Geometry: final body of the model. Coordinates: model frame, mm. A direction names the side the tool comes from. Coordinates: 2 decimals unless noted, no trailing zeros. Order: outer loops, then holes, each group sorted by start corner. A loop starts at its lowest first (then second) coordinate and runs counter-clockwise, first axis right, second up. Notation, with made-up numbers: (8, 86) -> (54, 86) arc R15 cw to (54, 90) -> close; hole circle Ø2 at (0.5, -33.5). An arc over 180 degrees is marked (long way). Use one line per item in the form item = value.
```python
from build123d import *

# Parameters (mm, degrees)
SKETCH1_W           = 150
SKETCH1_H           = 140
SKETCH1_R           = 2.85
SKETCH1_R_2         = 4
BOSS_EXTRUDE1_DEPTH = 5
SKETCH2_W           = 32
SKETCH2_H           = 18
SKETCH2_R           = 4
BOSS_EXTRUDE2_DEPTH = 5


with BuildPart() as part:
    # Sketch1 → Boss-Extrude1 (new body)
    with BuildSketch(Plane(origin=(0, 0, 0), x_dir=(1, 0, 0), z_dir=(0, 1, 0))):
        with Locations((-0.545997502, 48.457242913)):
            Rectangle(SKETCH1_W, SKETCH1_H)
        with Locations(Location((-65.545997502, 108.457242913, 0), (0, 0, 270))):
            Circle(SKETCH1_R, mode=Mode.SUBTRACT)
        with Locations(Location((64.454002498, 108.457242913, 0), (0, 0, 270))):
            Circle(SKETCH1_R, mode=Mode.SUBTRACT)
        with Locations(Location((64.454002498, -11.542757087, 0), (0, 0, 270))):
            Circle(SKETCH1_R, mode=Mode.SUBTRACT)
        with Locations(Location((-65.545997502, -11.542757087, 0), (0, 0, 270))):
            Circle(SKETCH1_R, mode=Mode.SUBTRACT)
        with Locations(Location((-11.545997502, 48.457242913, 0), (0, 0, 270))):
            Circle(SKETCH1_R_2, mode=Mode.SUBTRACT)
        with Locations(Location((-0.545997502, 48.457242913, 0), (0, 0, 270))):
            Circle(SKETCH1_R_2, mode=Mode.SUBTRACT)
        with Locations(Location((10.454002498, 48.457242913, 0), (0, 0, 270))):
            Circle(SKETCH1_R_2, mode=Mode.SUBTRACT)
    extrude(amount=BOSS_EXTRUDE1_DEPTH)

    # Sketch2 → Boss-Extrude2 (add)
    with BuildSketch(Plane(origin=(0, 5, 0), x_dir=(1, 0, 0), z_dir=(0, 1, 0))):
        with Locations((-0.545997502, 48.457242913)):
            Rectangle(SKETCH2_W, SKETCH2_H)
        with Locations(Location((-0.545997502, 48.457242913, 0), (0, 0, 270))):
            Circle(SKETCH2_R, mode=Mode.SUBTRACT)
        with Locations(Location((10.454002498, 48.457242913, 0), (0, 0, 270))):
            Circle(SKETCH2_R, mode=Mode.SUBTRACT)
        with Locations(Location((-11.545997502, 48.457242913, 0), (0, 0, 270))):
            Circle(SKETCH2_R, mode=Mode.SUBTRACT)
    extrude(amount=BOSS_EXTRUDE2_DEPTH)


solid = part.part
```
1) Section D-D, the plane z = -35.5. Output: boundary loops of the cut face in (x, y).
Results found:
outline = (-75.55, 0) -> (74.45, 0) -> (74.45, 5) -> (-75.55, 5) -> close
2) Pull-direction query (X, two-part tool) for faces 1 (the flat face through (74.454, 2, -47)), 2 (the flat face through (-2, 2, -118.457)), 3 (the cylindrical face through (-2.078, 4.93, -44.762)); classes: released by +X, released by -X, zero draft, split by the parting line, or undercut.
Results found:
face_1 = released by +X
face_2 = zero draft
face_3 = undercut
3) Contact query for flat-ended pins moving along their axis: P1, Ø6, axis at x = -25, z = -101, coming from the +Y side; P2, Ø1.5, axis at x = -1, y = 7, coming from the -Z side; P3, Ø4, axis at x = 2, y = 8.5, coming from the +Z side. Output: stop coordinate, or through.
Results found:
P1 = 5
P2 = -57.46
P3 = -39.46
4) Section C-C, the plane x = -34. Output: boundary loops of the cut face in (y, z), and give its area (3 significant figures).
Results found:
outline = (0, -118.46) -> (5, -118.46) -> (5, 21.54) -> (0, 21.54) -> close
area = 700 mm2
5) Access query for faces 4 (the cylindrical face through (-63.62, 2.46, -110.56)), 5 (the flat face through (-1, 7, -57.457)), 6 (the flat face through (-16.546, 7, -48)), 7 (the flat face through (-1, 7, -39.457)), 8 (the flat face through (15.454, 7, -48)). Directions: +Z, -Z, +X, -X, +Y, -Y. A direction counts if a zero-diameter tool reaches every point of the face in a straight line with its end or side. Return the directions, or none.
Results found:
face_4 = +Y, -Y
face_5 = -Z, +X, -X, +Y
face_6 = +Z, -Z, -X, +Y
face_7 = +Z, +X, -X, +Y
face_8 = +Z, -Z, +X, +Y
6) Section A-A, the plane y = 8.25. Output: boundary loops of the cut face in (x, z).
Results found:
outline = (-16.55, -57.46) -> (15.45, -57.46) -> (15.45, -39.46) -> (-16.55, -39.46) -> close; hole circle Ø8 at (-11.55, -48.46); hole circle Ø8 at (-0.55, -48.46); hole circle Ø8 at (10.45, -48.46)
7) Material intervals for probe 1 along Z at (x, y) = (-65, 2.75); probe 2 along Y at (x, z) = (-54, -5); probe 3 along Z at (x, y) = (5.5, 7.5), sorted ascending. Write a range as from..to.
Results found:
probe_1 = -118.46..-111.25, -105.66..8.75, 14.34..21.54
probe_2 = 0..5
probe_3 = -57.46..-39.46
8) Section B-B, the plane z = -54.5. Output: boundary loops of the cut face in (x, y), and give its area (3 significant figures).
Results found:
outline = (-75.55, 0) -> (74.45, 0) -> (74.45, 5) -> (15.45, 5) -> (15.45, 10) -> (-16.55, 10) -> (-16.55, 5) -> (-75.55, 5) -> close
area = 910 mm2
